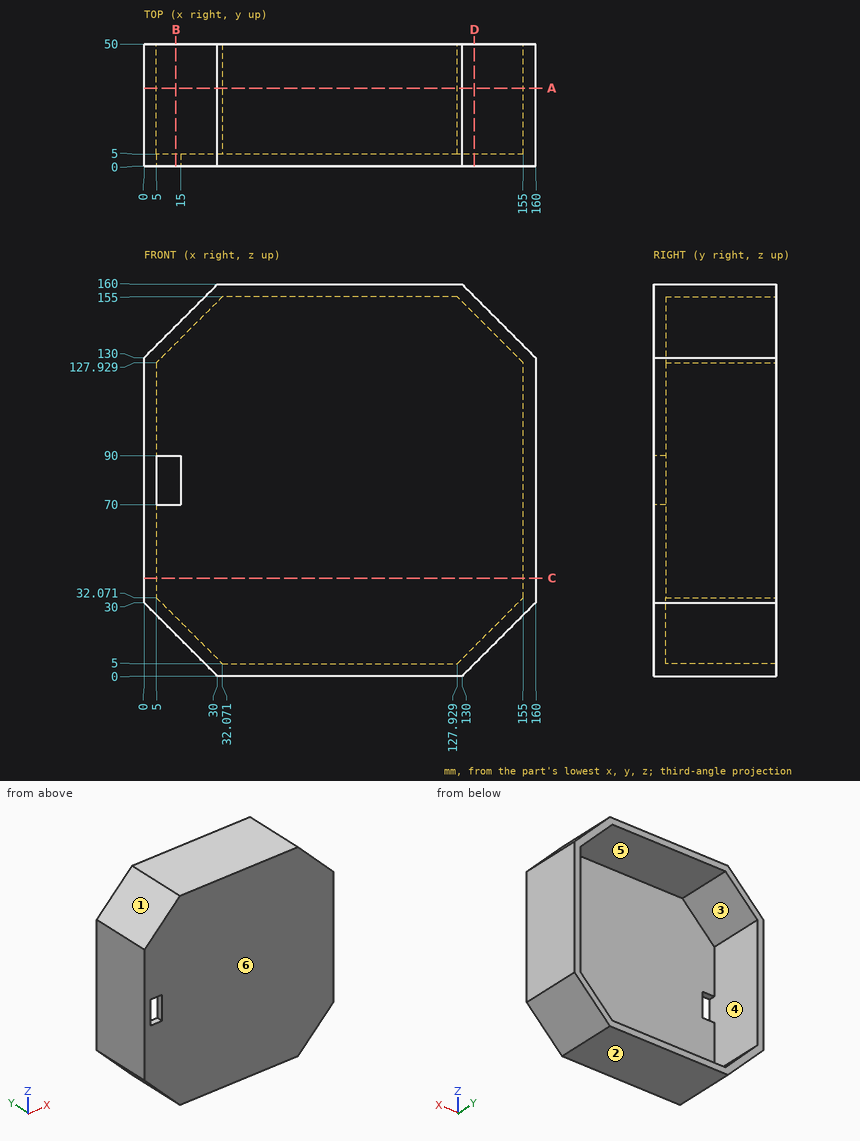
Input: dimensioned drawing with shaded views. Units: mm. Origin: part minimum x, y, z. A direction names the side the tool comes from. Round coordinates to 2 decimals unless told otherwise and drop trailing zeros. Order: outer loops, then holes, each group sorted by start corner. A loop starts at its lowest first (then second) coordinate and runs counter-clockwise, first axis right, second up.
1. Pin query (flat end, axial travel): P1, Ø1.5, axis at x = 80, y = 34, coming from the -Z side; P2, Ø12, axis at x = 113, z = 34, coming from the +Y side; P3, Ø5.5, axis at x = 9, y = 2, coming from the +Z side; P4, Ø1.5, axis at x = 12, y = 2.5, coming from the -Z side. Return the tip coordinate at first contact, or that it passes through.
The answers:
P1: stops at z = 0
P2: stops at y = 5
P3: stops at z = 141.75
P4: stops at z = 17.25
2. Cut plane C-C, the plane z = 40. Output: boundary loops of the cut face in (x, y), then the cut area to 3 significant figures.
The answers:
outline: (0, 0) - (160, 0) - (160, 50) - (155, 50) - (155, 5) - (5, 5) - (5, 50) - (0, 50) - close
area: 1,250 mm2
3. Set-up query: the marked faces 5 and 6. Return all of +Z, -Z, +X, -X, +Y, -Y with unobstructed straight access to the full face (end or side cutting, diameter ignored); none if empty.
The answers:
face 5: +Y
face 6: +Z, -Z, +X, -X, -Y
4. Cut plane D-D, the plane x = 135. Output: boundary loops of the cut face in (y, z).
The answers:
outline: (0, 5) - (50, 5) - (50, 12.07) - (5, 12.07) - (5, 147.93) - (50, 147.93) - (50, 155) - (0, 155) - close
5. Cut plane B-B, the plane x = 13. Output: boundary loops of the cut face in (y, z), then the cut area to 3 significant figures.
The answers:
outline: (0, 17) - (50, 17) - (50, 24.07) - (5, 24.07) - (5, 70) - (0, 70) - close; (0, 90) - (5, 90) - (5, 135.93) - (50, 135.93) - (50, 143) - (0, 143) - close
area: 1,170 mm2
6. Mould query, pull axis X, two halves, no side actions, for the marked faces 1, 2, 3 and 4. Classes: released by +X, released by -X, zero draft, split by the parting line, or undercut.
The answers:
face 1: released by -X
face 2: zero draft
face 3: undercut
face 4: undercut
7. Cut plane A-A, the plane y = 32. Output: boundary loops of the cut face in (x, z), then the cut area to 3 significant figures.
The answers:
outline: (0, 30) - (30, 0) - (130, 0) - (160, 30) - (160, 130) - (130, 160) - (30, 160) - (0, 130) - close; hole (5, 32.07) - (32.07, 5) - (127.93, 5) - (155, 32.07) - (155, 127.93) - (127.93, 155) - (32.07, 155) - (5, 127.93) - close
area: 2,770 mm2
8. Material intervals for line 1 (Z direction, x = 126.5, y = 24); line 2 (Y direction, x = 18.5, z = 133), sorted ascending.
The answers:
line 1: z = 0 to 5, 155 to 160
line 2: y = 0 to 5
